```python
from build123d import *

# Parameters (mm, degrees)
EXTRUDE_1_DEPTH             = 5
SKETCH_2_R                  = 1.6
CUT_EXTRUDE_1_DEPTH         = 22.794494718
HOLE_WIZARD_M41_D           = 4.2
HOLE_WIZARD_M41_DEPTH       = 8.5
HOLE_WIZARD_M41_CSINK_D     = 9.4
HOLE_WIZARD_M41_CSINK_ANGLE = 90
HOLE_WIZARD_M41_TIP         = 1.2618073
CUT_EXTRUDE_2_DEPTH         = 2.6


with BuildPart() as part:
    # Эскиз1 → Бобышка-Вытянуть1 (new body)
    with BuildSketch(Plane.XY):
        with BuildLine():
            Line((-15, 15), (15, 15))
            Line((15, 15), (15, 0))
            ThreePointArc((15, 0), (0, -15), (-15, 0))
            Line((-15, 0), (-15, 15))
        make_face()
    extrude(amount=EXTRUDE_1_DEPTH)

    # Эскиз2 → Вырез-Вытянуть1 (cut, through all)
    with BuildSketch(Plane.XY.offset(5)):
        with Locations((0, 10)):
            Circle(SKETCH_2_R)
        with Locations((8.660254038, -5)):
            Circle(SKETCH_2_R)
        with Locations((-8.660254038, -5)):
            Circle(SKETCH_2_R)
    extrude(amount=-CUT_EXTRUDE_1_DEPTH, mode=Mode.SUBTRACT)

    # Зенковка для винта с полупотайной головкой M41
    with Locations(Plane(origin=(-10, 5, 5), x_dir=(1, 0, 0), z_dir=(0, 0, 1))):
        with Locations((0, 0), (20, 0)):
            CounterSinkHole(HOLE_WIZARD_M41_D / 2, HOLE_WIZARD_M41_CSINK_D / 2, depth=HOLE_WIZARD_M41_DEPTH, counter_sink_angle=HOLE_WIZARD_M41_CSINK_ANGLE)
            with Locations((0, 0, -(HOLE_WIZARD_M41_DEPTH + HOLE_WIZARD_M41_TIP / 2))):  # 118° drill point
                Cone(0, HOLE_WIZARD_M41_D / 2, HOLE_WIZARD_M41_TIP, mode=Mode.SUBTRACT)

    # Эскиз4 → Вырез-Вытянуть2 (cut)
    with BuildSketch(Plane(origin=(0, 0, 0), x_dir=(-1, 0, 0), z_dir=(0, 0, -1))):
        Polygon((3.233161507, 10), (1.616580754, 12.8), (-1.616580754, 12.8), (-3.233161507, 10), (-1.616580754, 7.2), (1.616580754, 7.2), align=None)
        Polygon((11.893415545, -5), (10.276834792, -2.2), (7.043673284, -2.2), (5.42709253, -5), (7.043673284, -7.8), (10.276834792, -7.8), align=None)
        Polygon((-5.42709253, -5), (-7.043673284, -2.2), (-10.276834792, -2.2), (-11.893415545, -5), (-10.276834792, -7.8), (-7.043673284, -7.8), align=None)
    extrude(amount=-CUT_EXTRUDE_2_DEPTH, mode=Mode.SUBTRACT)


solid = part.part
```
Part model, mm, in its own coordinate system. A direction names the side the tool comes from. Give positions to 0.01 mm unless a question says otherwise; leave off trailing zeros. Write each loop counter-clockwise with the first axis right and the second up, starting at its lowest first coordinate (ties: lowest second). Pieces come first, ordered by that corner, then holes. Notation, with made-up numbers: (41, -21) -> (58, -21) arc R16 ccw to (58, -3) -> close; hole circle Ø2 at (-32.5, -17.75). An arc over 180 degrees is marked (long way). Put each result on its own line as item: value. Start each with the question number.
Item 1: Cut at A-A (z = 1.7). List the corners of the cut face in (x, y).
Item 2: Which spindle directions (+Z, -Z, +X, -X, +Y, -Y) get a long thin tool onto all of the face, cutting with end or side? Do faces 1 (the face through (-0.35, 8.44, 3.82)), 2 (the face through (-6.224, -6.38, 1.282)). Say none if no direction does.
Item 3: Cut at D-D (y = -9). List the corners of the cut face in (x, z).
Item 4: Wall check: L1, parallel to X at y = 5, z = 1.85; L2, parallel to Y at x = 0, z = 3.85; L3, parallel to X at y = 5.25, z = 3.8. Give the ranges that are in metal, low to high. Write a range as [from, to].
Item 5: Cut at B-B (x = 0). List the corners of the cut face in (y, z).
Item 6: Cut at C-C (z = 3.7). List the corners of the cut face in (x, y), then the cut area to 3 significant figures.
Item 7: Pin check, flat tips, straight feed: pin 1 Ø1.5 at (x, z) = (-8, 0.5) entering from -Y; pin 2 Ø0.8 at (x, z) = (-8, 1) entering from -Y; pin 3 Ø3 at (x, z) = (8.5, 2) entering from -Y. Stop position of each tip, or through.
Item 8: Pull direction X, two halves, no side cores. Call faces 3 (the face through (15, 8, 2)), 4 (the face through (10.186, -4.519, 3.817)), 5 (the face through (0, 15, 2)): pulls with the +X half, pulls with the -X half, needs draft (parallel to the pull), parting line crosses it, or undercut.
Answer list:
1. outline: (-15, 0) arc R15 ccw to (15, 0) -> (15, 15) -> (-15, 15) -> close; hole circle Ø4.2 at (-10, 5); hole (-11.89, -5) -> (-10.28, -7.8) -> (-7.04, -7.8) -> (-5.43, -5) -> (-7.04, -2.2) -> (-10.28, -2.2) -> close; hole (-3.23, 10) -> (-1.62, 7.2) -> (1.62, 7.2) -> (3.23, 10) -> (1.62, 12.8) -> (-1.62, 12.8) -> close; hole (5.43, -5) -> (7.04, -7.8) -> (10.28, -7.8) -> (11.89, -5) -> (10.28, -2.2) -> (7.04, -2.2) -> close; hole circle Ø4.2 at (10, 5)
2. face 1: +Z, -Z
2. face 2: -Z
3. outline: (-12, 0) -> (12, 0) -> (12, 5) -> (-12, 5) -> close
4. L1: x = [-15, -12.1], [-7.9, 7.9], [12.1, 15]
4. L2: y = [-15, 8.4], [11.6, 15]
4. L3: x = [-15, -13.49], [-6.51, 6.51], [13.49, 15]
5. outline: (-15, 0) -> (7.2, 0) -> (7.2, 2.6) -> (8.4, 2.6) -> (8.4, 5) -> (-15, 5) -> close; (11.6, 2.6) -> (12.8, 2.6) -> (12.8, 0) -> (15, 0) -> (15, 5) -> (11.6, 5) -> close
6. outline: (-15, 0) arc R15 ccw to (15, 0) -> (15, 15) -> (-15, 15) -> close; hole circle Ø6.8 at (-10, 5); hole circle Ø3.2 at (-8.66, -5); hole circle Ø3.2 at (0, 10); hole circle Ø6.8 at (10, 5); hole circle Ø3.2 at (8.66, -5)
6. area: 707 mm2
7. pin 1: stops at y = -13.13
7. pin 2: stops at y = -12.93
7. pin 3: stops at y = -13.27
8. face 3: pulls with the +X half
8. face 4: undercut
8. face 5: needs draft
